```python
from build123d import *

# Parameters (mm, degrees)
F0_R     = 1.15
F1_DEPTH = 4
F2_R     = 1.5
F3_DEPTH = 5
F4_R     = 1.5


with BuildPart() as f1:
    # F0 (on Front) → F1 (new body)
    with BuildSketch(Plane.XZ):
        with BuildLine():
            Line((5, -3.1), (5, 3.1))
            Line((5, 3.1), (-3.5, 3.1))
            ThreePointArc((-3.5, 3.1), (-3.93934, 2.03934), (-5, 1.6))
            Line((-5, 1.6), (-5, -1.6))
            ThreePointArc((-5, -1.6), (-3.93934, -2.03934), (-3.5, -3.1))
            Line((-3.5, -3.1), (5, -3.1))
        make_face()
        with Locations((2.5, 0)):
            Circle(F0_R, mode=Mode.SUBTRACT)
    extrude(amount=F1_DEPTH)

    # F2 (on face) → F3 (cut)
    with BuildSketch(Plane(origin=(-5, 0, 0), x_dir=(0, -1, 0), z_dir=(-1, 0, 0))):
        with Locations((2, 0)):
            Circle(F2_R)
    extrude(amount=-F3_DEPTH, mode=Mode.SUBTRACT)

    # F4
    f4_edges = [f1.edges().sort_by_distance(p)[0] for p in [
        (-3.5, -2, 3.1),
        (-3.5, -2, -3.1),
        (5, -2, 3.1),
        (5, -2, -3.1),
    ]]
    fillet(f4_edges, radius=F4_R)


solid = f1.part
```
Could you check a few things on this model? Use its own coordinates, in mm. A direction names the side the tool comes from. Coordinates: 2 decimals unless noted, no trailing zeros. Write each loop counter-clockwise with the first axis right and the second up, starting at its lowest first coordinate (ties: lowest second). Pieces come first, ordered by that corner, then holes. Notation, with made-up numbers: (-38.5, -39) -> (-17.5, -39) arc R19 cw to (-17.5, -35) -> close; hole circle Ø11 at (27.5, 25.5). An arc over 180 degrees is marked (long way). Return JSON: item names as keys, results as strings.
(1) Imagine slicing it at B-B, the plane y = -0.4. Please give me the cut outline in (x, z), then the cut area to 3 significant figures.
Numbers:
{"outline": "(-5, -1.6) arc R1.5 cw to (-3.7, -2.35) arc R1.5 ccw to (-2.4, -3.1) -> (3.5, -3.1) arc R1.5 ccw to (5, -1.6) -> (5, 1.6) arc R1.5 ccw to (3.5, 3.1) -> (-2.4, 3.1) arc R1.5 ccw to (-3.7, 2.35) arc R1.5 cw to (-5, 1.6) -> close; hole circle Ø2.3 at (2.5, 0)", "area": "53.0 mm2"}
(2) Which directions (+Z, -Z, +X, -X, +Y, -Y) give clear straight access to the entire face, cutting with the end or side of a thin tool? Please do faces 5 (the cylindrical face through (-2.54, -0.5, 0.07)), 6 (the flat face through (-5, -1.1, 1.4)).
Numbers:
{"face 5": "-X", "face 6": "+Z, -Z, -X, +Y, -Y"}
(3) I'm going to push flat-ended pins straight in: pin 1 (1.8 mm diameter, centred on x = 2.5, z = 0, fed in from -Y); pin 2 (1.8 mm diameter, centred on y = -2, z = 0, fed in from -X). Where does each tip first touch, or does it pass through?
Numbers:
{"pin 1": "passes through", "pin 2": "stops at x = 0"}
(4) Imagine slicing it at A-A, the plane x = 2.5. Please give me the cut outline in (y, z), then the cut area to 3 significant figures.
Numbers:
{"outline": "(-4, -3.1) -> (0, -3.1) -> (0, -1.15) -> (-4, -1.15) -> close; (-4, 1.15) -> (0, 1.15) -> (0, 3.1) -> (-4, 3.1) -> close", "area": "15.6 mm2"}
(5) Imagine slicing it at C-C, the plane z = 0. Please give me the cut outline in (x, y), then the cut area to 3 significant figures.
Numbers:
{"outline": "(-5, -4) -> (1.35, -4) -> (1.35, 0) -> (-5, 0) -> (-5, -0.5) -> (0, -0.5) -> (0, -3.5) -> (-5, -3.5) -> close; (3.65, -4) -> (5, -4) -> (5, 0) -> (3.65, 0) -> close", "area": "15.8 mm2"}
(6) Imagine slicing it at D-D, the plane x = -0.5. Please give me the cut outline in (y, z).
Numbers:
{"outline": "(-4, -3.1) -> (0, -3.1) -> (0, 3.1) -> (-4, 3.1) -> close; hole circle Ø3 at (-2, 0)"}
(7) I need wall thicknesses on L1, parallel to Z at x = -1, y = -2; L2, parallel to Z at x = 2.5, y = -3; L3, parallel to Y at x = -1.5, z = 0.25. Which ranges of each line are inside material? Lowest first, please.
Numbers:
{"L1": "z = -3.1 to -1.5, 1.5 to 3.1", "L2": "z = -3.1 to -1.15, 1.15 to 3.1", "L3": "y = -4 to -3.48, -0.52 to 0"}
(8) We'd pull the mould along Z, two halves only. Please class faces 1 (the flat face through (1, -2, 3.1)), 2 (the flat face through (0, -2, 0)), 3 (the flat face through (1, -2, -3.1)), 4 (the flat face through (0, 0, 0)): +Z half, -Z half, draft (parallel to the pull), parting line (faces both ways), or undercut.
Numbers:
{"face 1": "+Z half", "face 2": "undercut", "face 3": "-Z half", "face 4": "draft"}
